Source: CAD feature listing. Evaluate the final solid. Frame: model axes, mm. Face numbers are marked on the shaded views. A direction names the side the tool comes from. Coordinates: 2 decimals unless noted, no trailing zeros. Loops run counter-clockwise (first coordinate to the right, second up) from the corner with the lowest first, then second, coordinate; pieces in that order, holes last.
from build123d import *

# Parameters (mm, degrees)
F0_R     = 7.875
F0_R_2   = 2.25
F1_DEPTH = 7.5
F2_R     = 8.25
F2_R_2   = 2.75
F3_DEPTH = 7.5
F4_R     = 1.25
F5_DEPTH = 25


with BuildPart() as f1:
    # F0 (on Top) → F1 (new body)
    with BuildSketch(Plane.XY):
        Circle(F0_R)
        Circle(F0_R_2, mode=Mode.SUBTRACT)
    extrude(amount=F1_DEPTH)

    # F2 (on face) → F3 (join)
    with BuildSketch(Plane(origin=(0, 0, 0), x_dir=(1, 0, 0), z_dir=(0, 0, -1))):
        Circle(F2_R)
        Circle(F2_R_2, mode=Mode.SUBTRACT)
    extrude(amount=F3_DEPTH)

    # F4 (on Right) → F5 (cut)
    with BuildSketch(Plane.YZ):
        with Locations((0, 4.5)):
            Circle(F4_R)
        with Locations((0, -4.5)):
            Circle(F4_R)
    extrude(amount=-F5_DEPTH, mode=Mode.SUBTRACT)


solid = f1.part
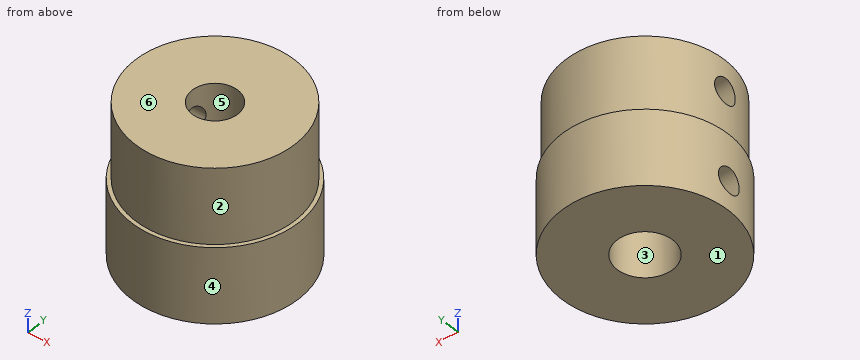
Q1. Draft query along X for the marked faces 3, 4, 5 and 6. Return one class per face: +X half, -X half, draft (parallel to the pull), parting line (faces both ways), or undercut.
Q2. Line query: line 1 along Y through (x, z) = (0, -3.75); line 2 along Y through (x, z) = (-6.25, 4.5); line 3 along X through (y, z) = (0, 3.75) (3 decimals). Output: solid intervals per line, ascending.
Q3. Contact query for flat-ended pins moving along their axis: pin 1 Ø6 at (y, z) = (5.5, -4.5) entering from -X; pin 2 Ø2 at (y, z) = (0, 4.5) entering from -X; pin 3 Ø8 at (x, z) = (-3.5, 5.5) entering from +Y (3 decimals). Output: stop coordinate, or through.
Q4. Section D-D, the plane y = 2.5. Return the cut outline in (x, z), plus the area to 3 significant figures.
Q5. Section A-A, the plane y = 0. Return the cut outline in (x, z) (3 decimals).
Q6. Section C-C, the plane z = 6.75. Return the cut outline in (x, y) (3 decimals).
Q7. Access query for the marked faces 1 and 2. Directions: +Z, -Z, +X, -X, +Y, -Y. A direction counts if a zero-diameter tool reaches every point of the face in a straight line with its end or side. Return the directions, or none.
Q8. Section B-B, the plane x = 0. Return the cut outline in (y, z) (3 decimals).
Derived:
1. face 3: undercut
1. face 4: parting line
1. face 5: undercut
1. face 6: draft
2. line 1: y = -8.25 to -2.75, 2.75 to 8.25
2. line 2: y = -4.79 to -1.25, 1.25 to 4.79
2. line 3: x = 2.25 to 7.875
3. pin 1: stops at x = -7.86
3. pin 2: stops at x = 2.02
3. pin 3: stops at y = 7.875
4. outline: (-7.86, -7.5) - (-1.15, -7.5) - (-1.15, 0) - (1.15, 0) - (1.15, -7.5) - (7.86, -7.5) - (7.86, 0) - (7.47, 0) - (7.47, 7.5) - (-7.47, 7.5) - (-7.47, 0) - (-7.86, 0) - close
4. area: 213 mm2
5. outline: (-8.25, -7.5) - (-2.75, -7.5) - (-2.75, -5.75) - (-8.25, -5.75) - close; (-8.25, -3.25) - (-2.75, -3.25) - (-2.75, 0) - (-2.25, 0) - (-2.25, 3.25) - (-7.875, 3.25) - (-7.875, 0) - (-8.25, 0) - close; (-7.875, 5.75) - (-2.25, 5.75) - (-2.25, 7.5) - (-7.875, 7.5) - close; (2.25, 0) - (2.75, 0) - (2.75, -7.5) - (8.25, -7.5) - (8.25, 0) - (7.875, 0) - (7.875, 7.5) - (2.25, 7.5) - close
6. outline: circle Ø15.75 at (0, 0); hole circle Ø4.5 at (0, 0)
7. face 1: -Z, +X, -X, +Y, -Y
7. face 2: +Z
8. outline: (-8.25, -7.5) - (-2.75, -7.5) - (-2.75, 0) - (-2.25, 0) - (-2.25, 7.5) - (-7.875, 7.5) - (-7.875, 0) - (-8.25, 0) - close; (2.25, 0) - (2.75, 0) - (2.75, -7.5) - (8.25, -7.5) - (8.25, 0) - (7.875, 0) - (7.875, 7.5) - (2.25, 7.5) - close
